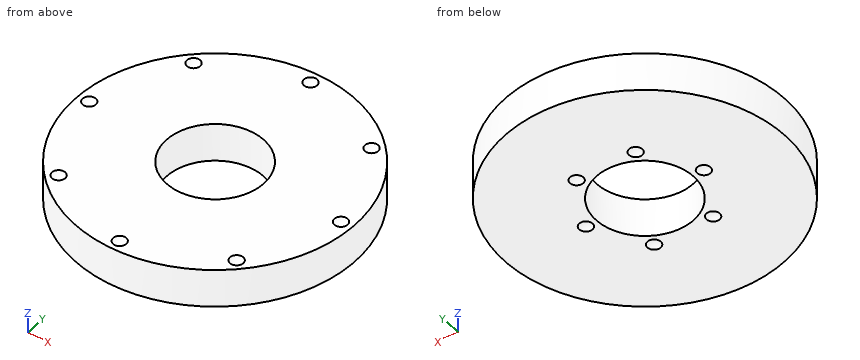
Autodesk Inventor part; units mm, degrees
ref_plane "YZ Plane" through (0, 0, 0) normal (1, 0, 0) x (0, 1, 0)
ref_plane "XZ Plane" through (0, 0, 0) normal (0, 1, 0) x (-1, 0, 0)
ref_plane "XY Plane" through (0, 0, 0) normal (0, 0, 1) x (1, 0, 0)
sketch "Sketch1" plane through (0, 0, 0) normal (0, 0, 1) x (1, 0, 0)
  circle A0 centre (0, 0) radius 6.35
  circle A1 centre (0, 0) radius 18.25
  dimension "d0" = 12.7
  dimension "d1" = 36.5
extrude "Extrusion1" add sketch "Sketch1" along normal blind 5
sketch "Sketch2" plane through (0, 0, 5) normal (0, 0, 1) x (1, 0, 0)
  circle A0 centre (0, 0) radius 6.35
  circle A1 centre (0, 0) radius 18.25
  circle A2 centre (0, 0) radius 7.1
  dimension "d4" = 14.2
sketch "Sketch3" plane through (0, 0, 0) normal (0, 1, 0) x (-1, 0, 0)
  line L0 (6.35, 0) -> (6.35, 5)
  line L1 (18.25, 0) -> (18.25, 5)
  line L2 (-18.25, 5) -> (18.25, 5)
  line L3 (-18.25, 0) -> (18.25, 0)
  line L4 (7.85, 5) -> (7.85, 0)
  line L5 (16.75, 5) -> (16.75, 0)
  line L6 (16.75, 5) -> (16.75, 7)
  line L7 (7.85, 5) -> (7.85, 8)
  line L8 (7.85, 0) -> (7.85, -2)
  circle A0 centre (16.75, 5.5) radius 1
  line L9 (16.75, 5) -> (16.75, 4.5)
  line L10 (16.75, 5) -> (15.884, 5)
  line L11 (16.75, 5) -> (17.616, 5)
  arc A1 (15.884, 5) -> (16.75, 4.5) centre (16.75, 5.5) ccw
  arc A2 (16.75, 4.5) -> (17.616, 5) centre (16.75, 5.5) ccw
  dimension "d5" = 1.5
  dimension "d6" = 1.5
  dimension "d9" = 0.5
  dimension "d10" = 2
revolve "Revolution1" cut sketch "Sketch3" angle 360 about axis through (-16.75, 0, 5) along (0, 0, -1) picked at (17.2864, 4.9436) contours L5 L2 A0
pattern_circular "Circular Pattern1" count 8 over 360 about axis through (0, 0, 0) along (0, 0, 1) of "Revolution1"
sketch "Sketch4" plane through (0, 0, 0) normal (0, 1, 0) x (-1, 0, 0)
  line L0 (18.25, 0) -> (18.25, 5)
  line L1 (6.35, 0) -> (6.35, 5)
  line L2 (-18.25, 0) -> (18.25, 0)
  line L3 (-18.25, 5) -> (18.25, 5)
  line L4 (7.85, 5) -> (7.85, 0)
  line L5 (7.85, 0) -> (7.85, -3)
  circle A0 centre (7.85, -0.5) radius 1
  line L6 (7.85, 0) -> (7.85, 0.5)
  line L7 (7.85, 0) -> (6.984, 0)
  line L8 (7.85, 0) -> (8.716, 0)
  arc A1 (8.716, 0) -> (7.85, 0.5) centre (7.85, -0.5) ccw
  arc A2 (7.85, 0.5) -> (6.984, 0) centre (7.85, -0.5) ccw
  dimension "d15" = 1.5
  dimension "d16" = 0.5
  dimension "d17" = 2
revolve "Revolution2" cut sketch "Sketch4" angle 360 about axis through (-7.85, 0, 5) along (0, 0, -1) picked at (8.3864, 0.0564) contours L2 L4 A0
pattern_circular "Circular Pattern2" count 6 over 360 about axis through (0, 0, 0) along (0, 0, 1) of "Revolution2"
properties part number "Plate between E2 and E3"
Input: part model. Units: mm. Frame: model coordinates. Coordinates: 2 decimals unless noted, no trailing zeros. Order: outer loops, then holes, each group sorted by start corner. A loop starts at its lowest first (then second) coordinate and runs counter-clockwise, first axis right, second up. Notation, with made-up numbers: M 43.25,60.25 L 78.25,60.25 A16 cw 78.25,78.25 Z; hole C 29,47 d11. An arc over 180 degrees is marked long. Write item = value, one per line. Start each with the question number.
(1) First-contact query: P1, Ø1.5, axis at x = -1, z = 3.5, coming from the +Y side; P2, Ø1, axis at y = 10.5, z = 2.5, coming from the -X side. Flat tips, straight axial feed; report the tip coordinate or a pass-through.
(2) Section C-C on z = 3.65. Output: boundary loops of the cut face in (x, y), and give its area (3 significant figures).
(3) Section D-D on x = -14.5. Output: boundary loops of the cut face in (y, z), and give its area (3 significant figures).
(4) Line query: line 1 along Y through (x, z) = (0, 3.7); line 2 along Y through (x, z) = (-4.5, 2); line 3 along Y through (x, z) = (-8, 4). Output: solid intervals per line, ascending. Write a range as [from, to].
(5) Section A-A on y = 0. Output: boundary loops of the cut face in (x, z), and give its area (3 significant figures).
(6) Section B-B on x = 0. Output: boundary loops of the cut face in (y, z), and give its area (3 significant figures).
Result set:
q1.P1 = 18.25
q1.P2 = -15.27
q2.outline = C 0,0 d36.5; hole C 0,0 d12.7
q2.area = 920 mm²
q3.outline = M -11.08,0 L 11.08,0 L 11.08,5 L -11.08,5 Z
q3.area = 111 mm²
q4.line_1 = [-18.25, -6.35], [6.35, 18.25]
q4.line_2 = [-17.69, -4.48], [4.48, 17.69]
q4.line_3 = [-16.4, 16.4]
q5.outline = M -18.25,0 L -8.72,0 A1 cw -6.98,0 L -6.35,0 L -6.35,5 L -15.88,5 A1 cw -17.62,5 L -18.25,5 Z; M 6.35,0 L 6.98,0 A1 cw 8.72,0 L 18.25,0 L 18.25,5 L 17.62,5 A1 cw 15.88,5 L 6.35,5 Z
q5.area = 117 mm²
q6.outline = M -18.25,0 L -6.35,0 L -6.35,5 L -15.88,5 A1 cw -17.62,5 L -18.25,5 Z; M 6.35,0 L 18.25,0 L 18.25,5 L 17.62,5 A1 cw 15.88,5 L 6.35,5 Z
q6.area = 118 mm²
